Autodesk Inventor part; units mm, degrees
ref_plane "YZ Plane" through (0, 0, 0) normal (1, 0, 0) x (0, 1, 0)
ref_plane "XZ Plane" through (0, 0, 0) normal (0, 1, 0) x (-1, 0, 0)
ref_plane "XY Plane" through (0, 0, 0) normal (0, 0, 1) x (1, 0, 0)
sketch "Sketch1" plane through (0, 0, 0) normal (0, 0, 1) x (1, 0, 0)
  line L0 (0, 17.6092) -> (15.25, -8.8046)
  line L1 (15.25, -8.8046) -> (-15.25, -8.8046)
  line L2 (-15.25, -8.8046) -> (0, 17.6092)
  circle A0 centre (-15.25, -8.8046) radius 2.25
  circle A1 centre (15.25, -8.8046) radius 2.25
  circle A2 centre (0, 17.6092) radius 2.25
  circle A3 centre (0, 0) radius 3.5
  circle A4 centre (-15.25, -8.8046) radius 6
  circle A5 centre (15.25, -8.8046) radius 6
  circle A6 centre (0, 17.6092) radius 6
  line L3 (5.1962, 20.6092) -> (20.4462, -5.8046)
  line L4 (15.25, -14.8046) -> (-15.25, -14.8046)
  line L5 (-20.4462, -5.8046) -> (-5.1962, 20.6092)
  dimension "d7" = 30.5
  dimension "d8" = 4.5
  dimension "d11" = 360
  dimension "d13" = 7
  dimension "d14" = 12
  dimension "d17" = 360
  dimension "d19" = 6
extrude "Extrusion1" add sketch "Sketch1" along normal blind 3.175 contours A2 L2 A6 L0 | L0 A6 L2 A2 | A6 L3 A5 L0 | L0 A5 L1 A4 L2 A6 | L2 A4 L5 A6 | A5 L1 A1 L0 | L0 A1 L1 A5 | A4 L1 A0 L2 | L2 A0 L1 A4 | A5 L4 A4 L1
sketch "Sketch2" plane through (0, 0, 0) normal (0, 0, -1) x (-1, 0, 0)
  circle A0 centre (0, 0) radius 3.5
  circle A1 centre (0, 0) radius 6.5
  circle A2 centre (0, 0) radius 3.5
  dimension "d22" = 13
extrude "Extrusion2" add sketch "Sketch2" along normal blind 4.5
fillet "Fillet1" radius 3 1 edges at (6.5, 0, 0)
sketch "Sketch3" plane through (0, 0, 3.175) normal (0, 0, 1) x (1, 0, 0)
  circle A0 centre (0, 0) radius 3.5
  line L0 (6.6973, 0) -> (3.3486, -5.8)
  line L1 (3.3486, -5.8) -> (-3.3486, -5.8)
  line L2 (-3.3486, -5.8) -> (-6.6973, 0)
  line L3 (-6.6973, 0) -> (-3.3486, 5.8)
  line L4 (-3.3486, 5.8) -> (3.3486, 5.8)
  line L5 (3.3486, 5.8) -> (6.6973, 0)
  circle A1 centre (0, 0) radius 9
  dimension "d26" = 11.6
  dimension "d27" = 18
extrude "Extrusion3" add sketch "Sketch3" along normal blind 4 contours A1
fillet "Fillet2" radius 2 1 edges at (-9, 0, 3.175)
properties part number "triangle_1"
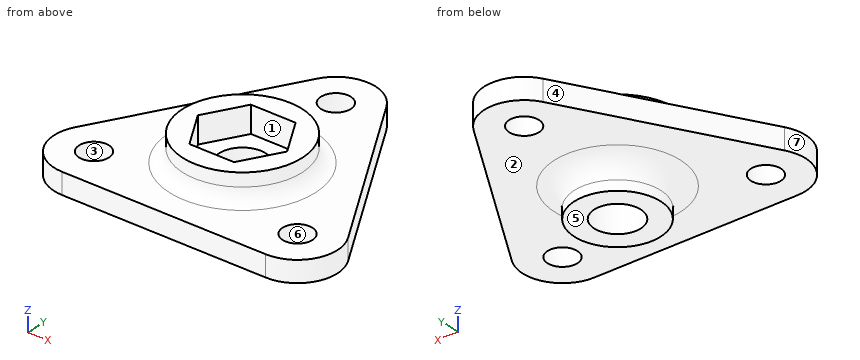
Could you check a few things on this model? Use its own coordinates, in mm. Face numbers are marked on the shaded views. A direction names the side the tool comes from. Coordinates: 2 decimals unless noted, no trailing zeros. Order: outer loops, then holes, each group sorted by start corner. A loop starts at its lowest first (then second) coordinate and runs counter-clockwise, first axis right, second up. Notation, with made-up numbers: (27, 26) - (34, 26) arc R8 ccw to (34, 31) - close; hole circle Ø1 at (-17.5, 28). An arc over 180 degrees is marked (long way). Answer in a Markdown table with one row per item. Add a question column.
(1) If we section it at B-B, the plane x = -13.5: Please give me the cut outline in (y, z) (3 decimals).
(2) If we section it at D-D, the plane z = -3.5: Please give me the cut outline in (x, y), then the cut area to 3 significant figures.
(3) I need wall thicknesses on L1, parallel to X at y = -7.5, z = 2; L2, parallel to Y at x = 0, z = -3.2; L3, parallel to Z at x = -19, y = -9.5 (3 decimals). Which ranges of each line are inside material? Lowest first, please.
(4) On a 3-axis mill with a long thin cutter (end or side, diameter ignored), from which of +Z, -Z, +X, -X, +Y, -Y can I reach the whole of each face in a straight line? I mean the marked faces 1, 2 and 3. Say none if no direction works.
(5) Will these pins go through, and if not, where does the flat tip stop? pin 1 (1 mm diameter, centred on x = 2.5, y = 13.5, fed in from -Z); pin 2 (6.5 mm diameter, centred on x = 0, y = 0, fed in from +Z); pin 3 (3 mm diameter, centred on x = -3, y = 13, fed in from +Z) (3 decimals); pin 4 (1.2 mm diameter, centred on x = 1.5, z = 6, fed in from -Y).
(6) If we section it at C-C, the plane y = 17: Please give me the cut outline in (x, z) (3 decimals), then the cut area to 3 significant figures.
(7) If we section it at A-A, the plane x = 0: Please give me the cut outline in (y, z) (3 decimals), then the cut area to 3 significant figures.
(8) If we mould it in two halves opening along Y, with no side actions, what happens to the marked faces 4, 5, 6 and 7? For each: released by +Y, released by -Y, zero draft, split by the parting line, or undercut.
Results are:
| question | item | result |
|---|---|---|
| 1 | outline | (-14.805, 0) - (-10.219, 0) - (-10.219, 3.175) - (-14.805, 3.175) - close; (-7.39, 0) - (6.227, 0) - (6.227, 3.175) - (-7.39, 3.175) - close |
| 2 | outline | circle Ø13 at (0, 0); hole circle Ø7 at (0, 0) |
| 2 | area | 94.2 mm2 |
| 3 | L1 | x = -21.11 to -17.08, -13.42 to 13.42, 17.08 to 21.11 |
| 3 | L2 | y = -6.5 to -3.5, 3.5 to 6.5 |
| 3 | L3 | z = 0 to 3.175 |
| 4 | face 1 | +Z |
| 4 | face 2 | -Z |
| 4 | face 3 | +Z, -Z |
| 5 | pin 1 | stops at z = 0 |
| 5 | pin 2 | passes through |
| 5 | pin 3 | stops at z = 3.175 |
| 5 | pin 4 | stops at y = -8.95 |
| 6 | outline | (-7.28, 0) - (-2.166, 0) - (-2.166, 3.175) - (-7.28, 3.175) - close; (2.166, 0) - (7.28, 0) - (7.28, 3.175) - (2.166, 3.175) - close |
| 6 | area | 32.5 mm2 |
| 7 | outline | (-14.805, 0) - (-9.5, 0) arc R3 cw to (-6.5, -3) - (-6.5, -4.5) - (-3.5, -4.5) - (-3.5, 3.175) - (-5.8, 3.175) - (-5.8, 7.175) - (-9, 7.175) - (-9, 5.175) arc R2 cw to (-11, 3.175) - (-14.805, 3.175) - close; (3.5, -4.5) - (6.5, -4.5) - (6.5, -3) arc R3 cw to (9.5, 0) - (15.359, 0) - (15.359, 3.175) - (11, 3.175) arc R2 cw to (9, 5.175) - (9, 7.175) - (5.8, 7.175) - (5.8, 3.175) - (3.5, 3.175) - close; (19.859, 0) - (23.609, 0) - (23.609, 3.175) - (19.859, 3.175) - close |
| 7 | area | 144 mm2 |
| 8 | face 4 | released by +Y |
| 8 | face 5 | zero draft |
| 8 | face 6 | undercut |
| 8 | face 7 | split by the parting line |
